Model file for the job. Use its own axes, mm. A direction names the side the tool comes from. Coordinates: 2 decimals unless noted, no trailing zeros. Order: outer loops, then holes, each group sorted by start corner. A loop starts at its lowest first (then second) coordinate and runs counter-clockwise, first axis right, second up.
from build123d import *

# Parameters (mm, degrees)
F0_R          = 12.7
F4_R          = 3.175
F5_DEPTH      = 25.4
F5_DEPTH_BACK = 25.4
F6_R          = 2.54


with BuildPart() as f2:
    # F2: sweep along a path in F1
    with BuildLine(Plane.XZ) as f2_path:
        Line((0, 304.8), (-177.8, 304.8))
        ThreePointArc((-177.8, 304.8), (-213.7210244843, 289.9210244843), (-228.6, 254))
        Line((-228.6, 254), (-228.6, 0))
    # F0 (on Top) → F2 (sweep)
    with BuildSketch(Plane.XY):
        with Locations((-228.6, 0)):
            Circle(F0_R)
    sweep(path=f2_path.line)

    # F3: F2 across plane


with BuildPart() as f2_1:
    add(f2.part)
    add(f2.part.mirror(Plane.YZ))

    # F4 (on Front) → F5 (cut, two sides)
    with BuildSketch(Plane.XZ) as f5_sk:
        with BuildLine():
            ThreePointArc((-228.6, 53.975), (-231.775, 50.8), (-228.6, 47.625))
            Line((-228.6, 47.625), (-228.6, 50.8))
            Line((-228.6, 50.8), (-228.6, 53.975))
        make_face()
        with BuildLine():
            ThreePointArc((-225.425, 177.8), (-230.8450640303, 180.0450640303), (-228.6, 174.625))
            ThreePointArc((-228.6, 174.625), (-226.3549359697, 175.5549359697), (-225.425, 177.8))
        make_face()
        with BuildLine():
            Line((-228.6, 50.8), (-228.6, 47.625))
            ThreePointArc((-228.6, 47.625), (-226.3549359697, 48.5549359697), (-225.425, 50.8))
            ThreePointArc((-225.425, 50.8), (-226.3549359697, 53.0450640303), (-228.6, 53.975))
            Line((-228.6, 53.975), (-228.6, 50.8))
        make_face()
        with Locations((228.6, 177.8)):
            Circle(F4_R)
        with Locations((228.6, 50.8)):
            Circle(F4_R)
    extrude(amount=F5_DEPTH, mode=Mode.SUBTRACT)
    extrude(f5_sk.sketch, amount=-F5_DEPTH_BACK, mode=Mode.SUBTRACT)

    # F6
    f6_edges = [f2_1.edges().sort_by_distance(p)[0] for p in [
        (241.3, 0, 0),
        (-241.3, 0, 0),
    ]]
    fillet(f6_edges, radius=F6_R)


solid = f2_1.part
Q1. Which spindle directions (+Z, -Z, +X, -X, +Y, -Y) get a long thin tool onto all of the face, cutting with end or side? Do faces 1 (the face through (216.486, -3.815, 126.51)), 2 (the face through (229, 0, 0)). Say none if no direction does.
Established:
face 1: -Z
face 2: -Z, +X, -X, +Y, -Y
Q2. Probe line 1 (X direction, y = -1.25, z = 29); line 2 (Z direction, x = -228.6, y = -9.75) (3 decimals); line 3 (Z direction, x = -228.6, y = 4) (3 decimals). List the from-to ranges inside material, lowest first.
Established:
line 1: x = -241.24 to -215.96, 215.96 to 241.24
line 2: z = 0 to 47.625, 53.975 to 174.625, 180.975 to 283.884
line 3: z = 0 to 47.625, 53.975 to 174.625, 180.975 to 291.013
Q3. Mould opens along X. For faces 3 (the face through (-216.486, -3.815, 126.51)), 4 (the face through (-229, 0, 0)) say: pulls with the +X half, pulls with the -X half, needs draft (parallel to the pull), parting line crosses it, or undercut.
Established:
face 3: undercut
face 4: needs draft
Q4. Cut at A-A, the plane z = 87.5. List the corners of the cut face in (x, y), plus the area to 3 significant figures.
Established:
outline: circle Ø25.4 at (-228.6, 0); circle Ø25.4 at (228.6, 0)
area: 1,010 mm2
Q5. Cut at B-B, the plane x = 10. List the corners of the cut face in (y, z), plus the area to 3 significant figures.
Established:
outline: circle Ø25.4 at (0, 304.8)
area: 507 mm2
Q6. Drop flat-ended pins along their axis: P1, Ø5.5, axis at x = 228.6, z = 50.8, coming from the -Y side; P2, Ø3, axis at y = 9, z = 200, coming from the +X side; P3, Ø10, axis at x = -133, y = 9.5, coming from the +Z side; P4, Ø1, axis at x = 44.5, y = -9, coming from the -Z side. Give the stop position or say it passes through.
Established:
P1: passes through
P2: stops at x = 238.85
P3: stops at z = 316.68
P4: stops at z = 295.36
